from build123d import *

# Parameters (mm, degrees)
SKETCH1_W           = 145
SKETCH1_H           = 95.6
BOSS_EXTRUDE1_DEPTH = 3.8
SKETCH2_W           = 131
SKETCH2_H           = 81.6
CUT_EXTRUDE1_DEPTH  = 174.720465116
FILLET1_R           = 10
SKETCH3_R           = 1
CUT_EXTRUDE2_DEPTH  = 174.720465116
SKETCH8_W           = 10
SKETCH8_H           = 3.8
CUT_EXTRUDE5_DEPTH  = 174.720465116
LPATTERN3_COUNT     = 4
LPATTERN3_PITCH     = 20
LPATTERN3_COL_COUNT = 4
LPATTERN3_COL_PITCH = 20
SKETCH9_W           = 3.8
SKETCH9_H           = 10
CUT_EXTRUDE6_DEPTH  = 174.720465116
LPATTERN4_COUNT     = 3
LPATTERN4_PITCH     = 20
LPATTERN4_COL_COUNT = 3
LPATTERN4_COL_PITCH = 20
SKETCH11_W          = 3.8
SKETCH11_H          = 10
SKETCH11_W_2        = 10
SKETCH11_H_2        = 3.8
BOSS_EXTRUDE4_DEPTH = 3.8


with BuildPart() as part:
    # Sketch1 → Boss-Extrude1 (new body)
    with BuildSketch(Plane(origin=(0, 0, 0), x_dir=(1, 0, 0), z_dir=(0, 1, 0))):
        with Locations((72.5, -47.8)):
            Rectangle(SKETCH1_W, SKETCH1_H)
    extrude(amount=BOSS_EXTRUDE1_DEPTH)

    # Sketch2 → Cut-Extrude1 (cut, through all)
    with BuildSketch(Plane(origin=(0, 3.8, 0), x_dir=(1, 0, 0), z_dir=(0, 1, 0))):
        with Locations((72.5, -47.8)):
            Rectangle(SKETCH2_W, SKETCH2_H)
    extrude(amount=-CUT_EXTRUDE1_DEPTH, mode=Mode.SUBTRACT)

    # Fillet1
    fillet1_edges = [part.edges().sort_by_distance(p)[0] for p in [
        (7, 1.9, 88.6),
        (7, 1.9, 7),
        (138, 1.9, 7),
        (138, 1.9, 88.6),
    ]]
    fillet(fillet1_edges, radius=FILLET1_R)

    # Sketch3 → Cut-Extrude2 (cut, through all)
    with BuildSketch(Plane.XZ):
        with Locations(Location((6.8, 88.8, 0), (0, 0, 270))):
            Circle(SKETCH3_R)
        with Locations(Location((138.2, 88.8, 0), (0, 0, 270))):
            Circle(SKETCH3_R)
        with Locations(Location((138.2, 6.8, 0), (0, 0, 270))):
            Circle(SKETCH3_R)
        with Locations(Location((6.8, 6.8, 0), (0, 0, 270))):
            Circle(SKETCH3_R)
    extrude(amount=-CUT_EXTRUDE2_DEPTH, mode=Mode.SUBTRACT)

    # Sketch8 → Cut-Extrude5 (cut, through all)
    with BuildSketch(Plane(origin=(0, 0, 0), x_dir=(-1, 0, 0), z_dir=(0, -1, 0))):
        with Locations((-72.5, -93.7)):
            Rectangle(SKETCH8_W, SKETCH8_H)
        with Locations((-72.5, -1.9)):
            Rectangle(SKETCH8_W, SKETCH8_H)
    cut_extrude5 = extrude(amount=-CUT_EXTRUDE5_DEPTH, mode=Mode.SUBTRACT)

    # LPattern3: Cut-Extrude5 ×4
    with Locations(*[(i * LPATTERN3_PITCH, 0, 0) for i in range(1, LPATTERN3_COUNT)]):
        add(cut_extrude5, mode=Mode.SUBTRACT)

    # LPattern3 col: Cut-Extrude5 ×4
    with Locations(*[(-i * LPATTERN3_COL_PITCH, 0, 0) for i in range(1, LPATTERN3_COL_COUNT)]):
        add(cut_extrude5, mode=Mode.SUBTRACT)

    # Sketch9 → Cut-Extrude6 (cut, through all)
    with BuildSketch(Plane(origin=(0, 0, 0), x_dir=(-1, 0, 0), z_dir=(0, -1, 0))):
        with Locations((-1.9, -47.8)):
            Rectangle(SKETCH9_W, SKETCH9_H)
        with Locations((-143.1, -47.8)):
            Rectangle(SKETCH9_W, SKETCH9_H)
    cut_extrude6 = extrude(amount=-CUT_EXTRUDE6_DEPTH, mode=Mode.SUBTRACT)

    # LPattern4: Cut-Extrude6 ×3
    with Locations(*[(0, 0, i * LPATTERN4_PITCH) for i in range(1, LPATTERN4_COUNT)]):
        add(cut_extrude6, mode=Mode.SUBTRACT)

    # LPattern4 col: Cut-Extrude6 ×3
    with Locations(*[(0, 0, -i * LPATTERN4_COL_PITCH) for i in range(1, LPATTERN4_COL_COUNT)]):
        add(cut_extrude6, mode=Mode.SUBTRACT)

    # Sketch11 → Boss-Extrude4 (add, through all)
    with BuildSketch(Plane(origin=(0, 0, 0), x_dir=(-1, 0, 0), z_dir=(0, -1, 0))):
        with Locations((-143.1, -87.8)):
            Rectangle(SKETCH11_W, SKETCH11_H)
        with Locations((-132.5, -93.7)):
            Rectangle(SKETCH11_W_2, SKETCH11_H_2)
        with Locations((-132.5, -1.9)):
            Rectangle(SKETCH11_W_2, SKETCH11_H_2)
        with Locations((-143.1, -7.8)):
            Rectangle(SKETCH11_W, SKETCH11_H)
        with Locations((-1.9, -7.8)):
            Rectangle(SKETCH11_W, SKETCH11_H)
        with Locations((-12.5, -1.9)):
            Rectangle(SKETCH11_W_2, SKETCH11_H_2)
        with Locations((-1.9, -87.8)):
            Rectangle(SKETCH11_W, SKETCH11_H)
        with Locations((-12.5, -93.7)):
            Rectangle(SKETCH11_W_2, SKETCH11_H_2)
    extrude(amount=-BOSS_EXTRUDE4_DEPTH)


solid = part.part
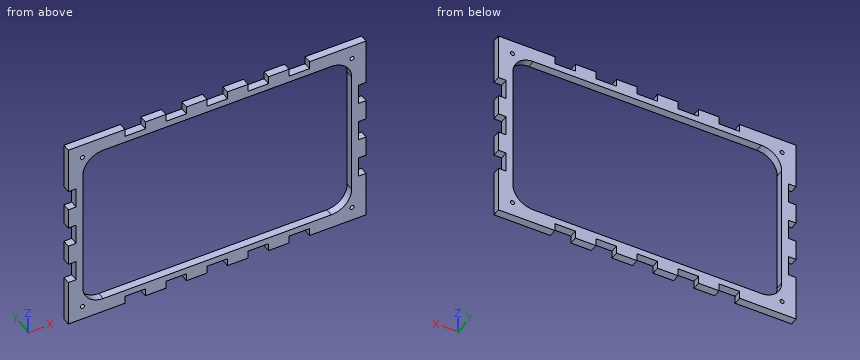
CAD build for the part. Positions are in the model's coordinates, mm. Coordinates: 2 decimals unless noted, no trailing zeros. Loops run counter-clockwise (first coordinate to the right, second up) from the corner with the lowest first, then second, coordinate; pieces in that order, holes last. Notation, with made-up numbers: (-2, -14.5) - (56, -14.5) arc R18 cw to (56, 16.5) - close; hole circle Ø11 at (32.5, 38). An arc over 180 degrees is marked (long way). Use one line per item in the form item = value. Start each with the question number.
1) Flat gauge pins, fed straight in: pin 1 (1.9 mm diameter, centred on x = 74.5, y = 1, fed in from -Z); pin 2 (1 mm diameter, centred on y = 2.5, z = 15, fed in from -X). Where does each tip first touch, or does it go through?
2) Band-saw the part on A-A (z = 50). Give the cut face in (x, y).
3) Band-saw the part on C-C (y = 0.75). State how many separate pieces and enclosed holes the cut face has, and give its area (3 significant figures).
4) Band-saw the part on B-B (x = 104). Give the cut face in (y, z).
5) Drill centre lines: L1, parallel to X at y = 2.6, z = 88.8; L2, parallel to Z at x = 138.2, y = 1.7; L3, parallel to Z at x = 122, y = 2.15. Where is each one in solid material? Low to high. Write a range as from..to.
Check values:
q1.pin_1 = 3.8
q1.pin_2 = 0
q2.outline = (3.8, 0) - (7, 0) - (7, 3.8) - (3.8, 3.8) - close; (138, 0) - (141.2, 0) - (141.2, 3.8) - (138, 3.8) - close
q3.separate_pieces = 1
q3.enclosed_holes = 5
q3.area = 2,640 mm2
q4.outline = (0, 0) - (3.8, 0) - (3.8, 7) - (0, 7) - close; (0, 88.6) - (3.8, 88.6) - (3.8, 95.6) - (0, 95.6) - close
q5.L1 = 0..5.8, 7.8..137.2, 139.2..145
q5.L2 = 0..5.8, 7.8..87.8, 89.8..95.6
q5.L3 = 0..7, 88.6..95.6
